Check sheet for the modelled part. Datum: model origin and axes. Units: mm. A direction names the side the tool comes from. Give positions to 0.01 mm unless a question says otherwise; leave off trailing zeros. Order: outer loops, then holes, each group sorted by start corner. A loop starts at its lowest first (then second) coordinate and runs counter-clockwise, first axis right, second up. Notation, with made-up numbers: (48.25, 5.5) -> (83.25, 5.5) arc R16 ccw to (83.25, 36.5) -> close; hole circle Ø3 at (43.5, 28). An arc over 180 degrees is marked (long way). One line per question, with ' | ' between items.
```python
from build123d import *

# Parameters (mm, degrees)
SKETCH1_W           = 25
SKETCH1_H           = 14.5
BOSS_EXTRUDE1_DEPTH = 9.5
CUT_EXTRUDE1_DEPTH  = 28.709429803
SKETCH3_W           = 11
SKETCH3_H           = 12.5
CUT_EXTRUDE2_DEPTH  = 18.293423606
SKETCH4_R           = 1.85
CUT_EXTRUDE3_DEPTH  = 19.406860134
FILLET1_R           = 2
SKETCH5_R           = 1.85
CUT_EXTRUDE4_DEPTH  = 21.06863224
SKETCH11_R          = 1.85
CUT_EXTRUDE10_DEPTH = 104.327776008


with BuildPart() as part:
    # Sketch1 → Boss-Extrude1 (new body)
    with BuildSketch(Plane.XY):
        Rectangle(SKETCH1_W, SKETCH1_H)
    extrude(amount=BOSS_EXTRUDE1_DEPTH)

    # Sketch2 → Cut-Extrude1 (cut, through all)
    with BuildSketch(Plane(origin=(12.5, 0, 0), x_dir=(0, 0, -1), z_dir=(1, 0, 0))):
        with BuildLine():
            Line((-9.5, 2.5), (-9.5, 8.25))
            Line((-9.5, 8.25), (0, 8.25))
            Line((0, 8.25), (0, 2.5))
            ThreePointArc((0, 2.5), (-4.75, 7.25), (-9.5, 2.5))
        make_face()
    extrude(amount=-CUT_EXTRUDE1_DEPTH, mode=Mode.SUBTRACT)

    # Sketch3 → Cut-Extrude2 (cut, through all)
    with BuildSketch(Plane.XY.offset(9.5)):
        with Locations((7, 1)):
            Rectangle(SKETCH3_W, SKETCH3_H)
        with Locations((-7, 1)):
            Rectangle(SKETCH3_W, SKETCH3_H)
    extrude(amount=-CUT_EXTRUDE2_DEPTH, mode=Mode.SUBTRACT)

    # Sketch4 → Cut-Extrude3 (cut, through all)
    with BuildSketch(Plane(origin=(1.5, 0, 0), x_dir=(0, 0, -1), z_dir=(1, 0, 0))):
        with Locations(Location((-4.75, 2.5, 0), (0, 0, 90))):
            Circle(SKETCH4_R)
    extrude(amount=-CUT_EXTRUDE3_DEPTH, mode=Mode.SUBTRACT)

    # Fillet1
    fillet1_edges = [part.edges().sort_by_distance(p)[0] for p in [
        (12.5, -6.25, 9.5),
        (12.5, -6.25, 0),
        (-12.5, -6.25, 9.5),
        (-12.5, -6.25, 0),
    ]]
    fillet(fillet1_edges, radius=FILLET1_R)

    # Sketch5 → Cut-Extrude4 (cut, through all)
    with BuildSketch(Plane(origin=(0, -5.25, 0), x_dir=(1, 0, 0), z_dir=(0, 1, 0))):
        with Locations(Location((-8, -4.75, 0), (0, 0, 180))):
            Circle(SKETCH5_R)
        with Locations(Location((8, -4.75, 0), (0, 0, 180))):
            Circle(SKETCH5_R)
    extrude(amount=-CUT_EXTRUDE4_DEPTH, mode=Mode.SUBTRACT)

    # Sketch11 → Cut-Extrude10 (cut, through all)
    with BuildSketch(Plane(origin=(-55.7, -5.25, -67.11030802), x_dir=(-1, 0, 0), z_dir=(0, 1, 0))):
        with Locations((-47.633605072, 71.30556155)):
            Circle(SKETCH11_R)
    extrude(amount=-CUT_EXTRUDE10_DEPTH, mode=Mode.SUBTRACT)


solid = part.part
```
Q1. Access from +Z, -Z, +X, -X, +Y, -Y to the whole of each face (thin tool, end or side, straight path). Record for faces 5 (the face through (6, -5.25, 5)), 6 (the face through (-7.82, -6.24, 6.59)), 7 (the face through (-1.5, 0, 5)).
Result sheet:
face 5: +Z, -Z, +X, +Y | face 6: +Y, -Y | face 7: +Z, -Z, -X, +Y
Q2. Thickness scan on line 1 (Z direction, x = 0.5, y = 2.5); line 2 (Y direction, x = 4.5, z = 9); line 3 (X direction, y = 6.5, z = 2.25). Record the ranges inside material, lowest first.
Result sheet:
line 1: z = 0 to 2.9, 6.6 to 9.5 | line 2: y = -7.25 to -5.25 | line 3: x = -1.5 to 1.5
Q3. Section check C-C (y = 1). Enter the section's corners in (x, z).
Result sheet:
outline: (-1.5, 0) -> (1.5, 0) -> (1.5, 3.67) -> (-1.5, 3.67) -> close; (-1.5, 5.83) -> (1.5, 5.83) -> (1.5, 9.5) -> (-1.5, 9.5) -> close
Q4. Section check D-D (z = 1.25). Enter the section's corners in (x, y).
Result sheet:
outline: (-12.35, -7.25) -> (12.35, -7.25) -> (12.35, -5.25) -> (1.5, -5.25) -> (1.5, 5.71) -> (-1.5, 5.71) -> (-1.5, -5.25) -> (-12.35, -5.25) -> close
Q5. Section check B-B (z = 5.5). Enter the section's corners in (x, y).
Result sheet:
outline: (-12.5, -7.25) -> (-9.69, -7.25) -> (-9.69, -5.25) -> (-12.5, -5.25) -> close; (-6.31, -7.25) -> (6.31, -7.25) -> (6.31, -5.25) -> (1.5, -5.25) -> (1.5, 0.81) -> (-1.5, 0.81) -> (-1.5, -5.25) -> (-6.31, -5.25) -> close; (-1.5, 4.19) -> (1.5, 4.19) -> (1.5, 7.19) -> (-1.5, 7.19) -> close; (9.69, -7.25) -> (12.5, -7.25) -> (12.5, -5.25) -> (9.69, -5.25) -> close
Q6. Mould release check, pull along Z, two halves, no side actions. Record for faces 1 (the face through (-11.93, -6.24, 0.6)), 2 (the face through (12.5, -6, 5)), 3 (the face through (0.02, 7.25, 4.65)), 4 (the face through (9.85, -6.24, 4.83)): pulls with the +Z half, pulls with the -Z half, needs draft (parallel to the pull), parting line crosses it, or undercut.
Result sheet:
face 1: pulls with the -Z half | face 2: needs draft | face 3: parting line crosses it | face 4: undercut
Q7. Section check A-A (x = 8). Enter the section's corners in (y, z).
Result sheet:
outline: (-7.25, 0) -> (-5.25, 0) -> (-5.25, 2.9) -> (-7.25, 2.9) -> close; (-7.25, 6.6) -> (-5.25, 6.6) -> (-5.25, 9.5) -> (-7.25, 9.5) -> close
Q8. Depth check by flat-ended pin: pin 1 Ø3 at (y, z) = (-0.5, 4.5) entering from +X; pin 2 Ø3 at (y, z) = (2.5, 4.75) entering from +X; pin 3 Ø5 at (x, z) = (9, 4) entering from +Y; pin 4 Ø3 at (x, z) = (-1.5, 3) entering from +Y. Enter the tip coordinate at first touch or a pass-through.
Result sheet:
pin 1: stops at x = 1.5 | pin 2: passes through | pin 3: stops at y = -5.25 | pin 4: stops at y = 7.24
